Could you check a few things on this model? Use its own coordinates, in mm. Face numbers are marked on the shaded views. A direction names the side the tool comes from. Round coordinates to 2 decimals unless told otherwise and drop trailing zeros. Loops run counter-clockwise (first coordinate to the right, second up) from the corner with the lowest first, then second, coordinate; pieces in that order, holes last. Notation, with made-up numbers: (-23.5, 80.5) - (-9.5, 80.5) arc R27 cw to (-9.5, 106.5) - close; hole circle Ø6 at (69.5, 23.5). An arc over 180 degrees is marked (long way). Put each result on its own line as item: value. Start each with the question number.
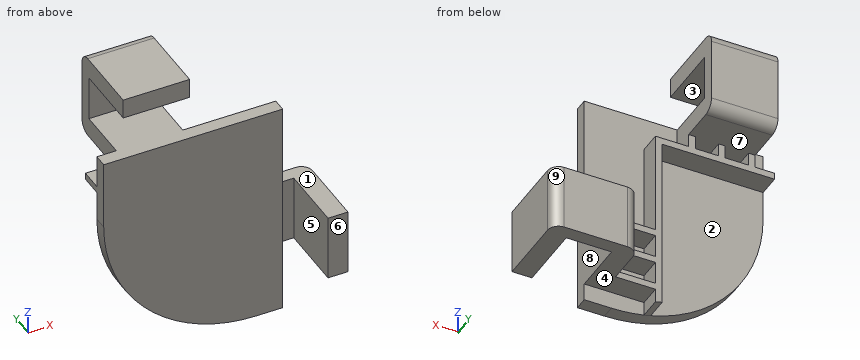
from build123d import *

# Parameters (mm, degrees)
SKETCH1_W           = 30
SKETCH1_H           = 9
SKETCH1_W_2         = 9
SKETCH1_H_2         = 30
BOSS_EXTRUDE1_DEPTH = 6
BOSS_EXTRUDE2_START = 6
SKETCH1_3_W         = 30
SKETCH1_3_H         = 9
SKETCH1_3_W_2       = 9
SKETCH1_3_H_2       = 30
BOSS_EXTRUDE2_DEPTH = 24
BOSS_EXTRUDE3_START = 30
SKETCH1_4_W         = 30
SKETCH1_4_H         = 9
SKETCH1_4_H_2       = 20.5
SKETCH1_4_W_2       = 9
SKETCH1_4_H_3       = 30
SKETCH1_4_W_3       = 20.5
BOSS_EXTRUDE3_DEPTH = 6
BOSS_EXTRUDE4_START = 30
SKETCH1_5_W         = 30
SKETCH1_5_H         = 9
SKETCH1_5_W_2       = 9
SKETCH1_5_H_2       = 30
BOSS_EXTRUDE4_DEPTH = 30
SKETCH2_W           = 3
SKETCH2_H           = 6
SKETCH2_W_2         = 18
SKETCH2_H_2         = 3
BOSS_EXTRUDE5_DEPTH = 10
FILLET1_R           = 5


with BuildPart() as part:
    # Sketch1 → Boss-Extrude1 (new body)
    with BuildSketch(Plane(origin=(0, 0, 0), x_dir=(1, 0, 0), z_dir=(0, 1, 0))):
        with Locations((-57, 4.5)):
            Rectangle(SKETCH1_W, SKETCH1_H)
        with Locations((-4.5, 77)):
            Rectangle(SKETCH1_W_2, SKETCH1_H_2)
        with BuildLine():
            Line((0, 99.896112213), (-12.24628833, 99.896112213))
            ThreePointArc((-12.24628833, 99.896112213), (-60.703064532, 79.824658322), (-80.774518424, 31.36788212))
            Line((-80.774518424, 31.36788212), (-80.774518424, 0))
            Line((-80.774518424, 0), (-72, 0))
            Line((-72, 0), (-72, 9))
            Line((-72, 9), (-42, 9))
            Line((-42, 9), (-42, 0))
            Line((-42, 0), (0, 0))
            Line((0, 0), (0, 62))
            Line((0, 62), (-9, 62))
            Line((-9, 62), (-9, 92))
            Line((-9, 92), (0, 92))
            Line((0, 92), (0, 99.896112213))
        make_face()
    extrude(amount=BOSS_EXTRUDE1_DEPTH)

    # Sketch1<3> → Boss-Extrude2 (add)
    with BuildSketch(Plane(origin=(0, 0, 0), x_dir=(1, 0, 0), z_dir=(0, 1, 0)).offset(BOSS_EXTRUDE2_START)):
        with Locations((-57, 4.5)):
            Rectangle(SKETCH1_3_W, SKETCH1_3_H)
        with Locations((-4.5, 77)):
            Rectangle(SKETCH1_3_W_2, SKETCH1_3_H_2)
    extrude(amount=BOSS_EXTRUDE2_DEPTH)

    # Sketch1<4> → Boss-Extrude3 (add)
    with BuildSketch(Plane(origin=(0, 0, 0), x_dir=(1, 0, 0), z_dir=(0, 1, 0)).offset(BOSS_EXTRUDE3_START)):
        with Locations((-57, 4.5)):
            Rectangle(SKETCH1_4_W, SKETCH1_4_H)
        with Locations((-57, -10.25)):
            Rectangle(SKETCH1_4_W, SKETCH1_4_H_2)
        with Locations((-57, -25)):
            Rectangle(SKETCH1_4_W, SKETCH1_4_H)
        with Locations((-4.5, 77)):
            Rectangle(SKETCH1_4_W_2, SKETCH1_4_H_3)
        with Locations((10.25, 77)):
            Rectangle(SKETCH1_4_W_3, SKETCH1_4_H_3)
        with Locations((25, 77)):
            Rectangle(SKETCH1_4_W_2, SKETCH1_4_H_3)
    extrude(amount=BOSS_EXTRUDE3_DEPTH)

    # Sketch1<5> → Boss-Extrude4 (add)
    with BuildSketch(Plane(origin=(0, 0, 0), x_dir=(1, 0, 0), z_dir=(0, 1, 0)).offset(BOSS_EXTRUDE4_START)):
        with Locations((-57, -25)):
            Rectangle(SKETCH1_5_W, SKETCH1_5_H)
        with Locations((25, 77)):
            Rectangle(SKETCH1_5_W_2, SKETCH1_5_H_2)
    extrude(amount=-BOSS_EXTRUDE4_DEPTH)

    # Sketch2 → Boss-Extrude5 (add)
    with BuildSketch(Plane(origin=(0, 6, 0), x_dir=(1, 0, 0), z_dir=(0, 1, 0))):
        with BuildLine():
            Line((-27, 89), (-27, 92))
            Line((-27, 92), (-27, 98.289076907))
            ThreePointArc((-27, 98.289076907), (-28.50412753, 97.9396553), (-30, 97.556431293))
            Line((-30, 97.556431293), (-30, 18))
            Line((-30, 18), (-80.774518424, 18))
            Line((-80.774518424, 18), (-80.774518424, 15))
            Line((-80.774518424, 15), (-72, 15))
            Line((-72, 15), (-69, 15))
            Line((-69, 15), (-58.5, 15))
            Line((-58.5, 15), (-55.5, 15))
            Line((-55.5, 15), (-45, 15))
            Line((-45, 15), (-42, 15))
            Line((-42, 15), (-27, 15))
            Line((-27, 15), (-27, 62))
            Line((-27, 62), (-27, 65))
            Line((-27, 65), (-27, 75.5))
            Line((-27, 75.5), (-27, 78.5))
            Line((-27, 78.5), (-27, 89))
        make_face()
        with Locations((-57, 12)):
            Rectangle(SKETCH2_W, SKETCH2_H)
        with Locations((-18, 77)):
            Rectangle(SKETCH2_W_2, SKETCH2_H_2)
        with Locations((-70.5, 12)):
            Rectangle(SKETCH2_W, SKETCH2_H)
        with Locations((-43.5, 12)):
            Rectangle(SKETCH2_W, SKETCH2_H)
        with Locations((-18, 63.5)):
            Rectangle(SKETCH2_W_2, SKETCH2_H_2)
        with Locations((-18, 90.5)):
            Rectangle(SKETCH2_W_2, SKETCH2_H_2)
    extrude(amount=BOSS_EXTRUDE5_DEPTH)

    # Fillet1
    fillet1_edges = [part.edges().sort_by_distance(p)[0] for p in [
        (-57, 36, -9),
        (-57, 36, 29.5),
        (29.5, 36, -77),
        (-9, 36, -77),
    ]]
    fillet(fillet1_edges, radius=FILLET1_R)


solid = part.part
Item 1: Thinking about a two-plate mould opening in X: for the marked faces 6, 7, 8 and 9, which applies, released by +X, released by -X, zero draft, split by the parting line, or undercut?
Item 2: Will these pins go through, and if not, where does the flat tip stop? P1, Ø1.8, axis at x = -49, z = -12, coming from the +Y side; P2, Ø1.9, axis at y = 12, z = -96, coming from the +X side; P3, Ø10, axis at y = 7.5, z = -56, coming from the -X side.
Item 3: Suppose I cut it at C-C, the plane z = -12.5. List the corners of the cut face in (x, y) for me, then the cut area to 3 significant figures.
Item 4: Suppose I cut it at D-D, the plane x = -20.5. List the corners of the cut face in (y, z) for me, then the cut area to 3 significant figures.
Item 5: Suppose I cut it at B-B, the plane y = 4. List the corners of the cut face in (x, z) for me.
Item 6: I need wall thicknesses on line 1 (Z direction, x = -20.5, y = 11.5); line 2 (X direction, y = 27, z = -72.5); line 3 (Y direction, x = -1.5, z = -53). Which ranges of each line are inside material? Lowest first, please. Write a range as from..to.
Item 7: Suppose I cut it at A-A, the plane y = 17.5. List the corners of the cut face in (x, z) for me, then the cut area to 3 significant figures.
Item 8: On a 3-axis mill with a long thin cutter (end or side, diameter ignored), from which of +Z, -Z, +X, -X, +Y, -Y can I reach the whole of each face in a straight line? I mean the marked faces 1, 2, 3, 4 and 5. Say none if no direction works.
Numbers:
1. face 6: zero draft
1. face 7: undercut
1. face 8: undercut
1. face 9: released by +X
2. P1: y = 6
2. P2: x = -27
2. P3: x = -77.83
3. outline: (-80.77, 0) - (0, 0) - (0, 6) - (-42, 6) - (-42, 16) - (-45, 16) - (-45, 6) - (-55.5, 6) - (-55.5, 16) - (-58.5, 16) - (-58.5, 6) - (-69, 6) - (-69, 16) - (-72, 16) - (-72, 6) - (-80.77, 6) - close
3. area: 575 mm^2
4. outline: (0, -99.4) - (6, -99.4) - (6, -92) - (16, -92) - (16, -89) - (6, -89) - (6, -78.5) - (16, -78.5) - (16, -75.5) - (6, -75.5) - (6, -65) - (16, -65) - (16, -62) - (6, -62) - (6, 0) - (0, 0) - close
4. area: 686 mm^2
5. outline: (-80.77, -31.37) arc R68.53 ccw to (-12.25, -99.9) - (0, -99.9) - (0, 0) - (-80.77, 0) - close; (-72, 20.5) - (-42, 20.5) - (-42, 29.5) - (-72, 29.5) - close; (20.5, -92) - (29.5, -92) - (29.5, -62) - (20.5, -62) - close
6. line 1: -92..-89, -78.5..-75.5, -65..-62
6. line 2: -9..0, 20.5..29.5
6. line 3: 0..6
7. outline: (-72, -9) - (-42, -9) - (-42, 0) - (-72, 0) - close; (-72, 20.5) - (-42, 20.5) - (-42, 29.5) - (-72, 29.5) - close; (-9, -92) - (0, -92) - (0, -62) - (-9, -62) - close; (20.5, -92) - (29.5, -92) - (29.5, -62) - (20.5, -62) - close
7. area: 1,080 mm^2
8. face 1: +Z, +X, +Y
8. face 2: -Z, -X, +Y
8. face 3: +X, -X, -Y
8. face 4: -Z, +X, +Y
8. face 5: +Z, -Z, -Y
